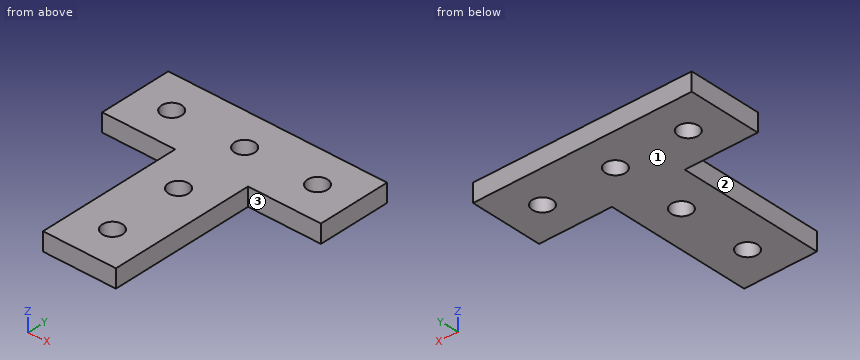
```python
from build123d import *

# Parameters (mm, degrees)
BOSS_EXTRUDE1_DEPTH = 6.35
SKETCH2_R           = 3.5
CUT_EXTRUDE1_DEPTH  = 7.35


with BuildPart() as part:
    # Sketch1 → Boss-Extrude1 (new body)
    with BuildSketch(Plane.XY):
        Polygon((12.7, 0), (-12.7, 0), (-12.7, 50.8), (-38.1, 50.8), (-38.1, 76.2), (38.1, 76.2), (38.1, 50.8), (12.7, 50.8), align=None)
    extrude(amount=BOSS_EXTRUDE1_DEPTH)

    # Sketch2 → Cut-Extrude1 (cut, through all)
    with BuildSketch(Plane.XY.offset(6.35)):
        with Locations((0, 63.5)):
            Circle(SKETCH2_R)
        with Locations((25.4, 63.5)):
            Circle(SKETCH2_R)
        with Locations((-25.4, 63.5)):
            Circle(SKETCH2_R)
        with Locations((0, 38.1)):
            Circle(SKETCH2_R)
        with Locations((0, 12.7)):
            Circle(SKETCH2_R)
    extrude(amount=-CUT_EXTRUDE1_DEPTH, mode=Mode.SUBTRACT)


solid = part.part
```
Read the model definition and answer for the solid it produces. Units are mm, in the model's axes. Face numbers are marked on the shaded views. A direction names the side the tool comes from. Coordinates: 2 decimals unless noted, no trailing zeros. Write each loop counter-clockwise with the first axis right and the second up, starting at its lowest first coordinate (ties: lowest second). Pieces come first, ordered by that corner, then holes. Notation, with made-up numbers: (-19.75, 43) -> (21.25, 43) arc R23 ccw to (21.25, 62) -> close; hole circle Ø5 at (-3.5, -34.5). An arc over 180 degrees is marked (long way). Answer as a JSON object with one key per item and string values.
Q1. Consider line 1 (Y direction, x = 0, z = 3.25); line 2 (Y direction, x = 25.4, z = 4.5); line 3 (X direction, y = 34.5, z = 3.75). Determine where each line is inside the solid, lowest interval first. Write a range as [from, to].
The answers:
{"line 1": "y = [0, 9.2], [16.2, 34.6], [41.6, 60], [67, 76.2]", "line 2": "y = [50.8, 60], [67, 76.2]", "line 3": "x = [-12.7, 12.7]"}
Q2. The part is cut by section B-B on y = 12.7. Give the vertices of the cut face in (x, z).
The answers:
{"outline": "(-12.7, 0) -> (-3.5, 0) -> (-3.5, 6.35) -> (-12.7, 6.35) -> close; (3.5, 0) -> (12.7, 0) -> (12.7, 6.35) -> (3.5, 6.35) -> close"}
Q3. The part is cut by section A-A on x = 25.4. Give the vertices of the cut face in (y, z).
The answers:
{"outline": "(50.8, 0) -> (60, 0) -> (60, 6.35) -> (50.8, 6.35) -> close; (67, 0) -> (76.2, 0) -> (76.2, 6.35) -> (67, 6.35) -> close"}
Q4. The part is cut by section D-D on y = 63.5. Give the vertices of the cut face in (x, z).
The answers:
{"outline": "(-38.1, 0) -> (-28.9, 0) -> (-28.9, 6.35) -> (-38.1, 6.35) -> close; (-21.9, 0) -> (-3.5, 0) -> (-3.5, 6.35) -> (-21.9, 6.35) -> close; (3.5, 0) -> (21.9, 0) -> (21.9, 6.35) -> (3.5, 6.35) -> close; (28.9, 0) -> (38.1, 0) -> (38.1, 6.35) -> (28.9, 6.35) -> close"}
Q5. Flat-ended cylindrical pins translate along their axes: pin 1 Ø6.5 at (x, y) = (0, 12.7) entering from +Z; pin 2 Ø1.9 at (y, z) = (26.5, 3) entering from -X; pin 3 Ø1.9 at (x, z) = (28.5, 4.5) entering from -Y; pin 4 Ø1.9 at (y, z) = (28, 2) entering from +X. Find the tip coordinate at first contact, or state that the pin passes through.
The answers:
{"pin 1": "passes through", "pin 2": "stops at x = -12.7", "pin 3": "stops at y = 50.8", "pin 4": "stops at x = 12.7"}
Q6. The part is cut by section C-C on z = 4.75. Give the vertices of the cut face in (x, y).
The answers:
{"outline": "(-38.1, 50.8) -> (-12.7, 50.8) -> (-12.7, 0) -> (12.7, 0) -> (12.7, 50.8) -> (38.1, 50.8) -> (38.1, 76.2) -> (-38.1, 76.2) -> close; hole circle Ø7 at (-25.4, 63.5); hole circle Ø7 at (0, 12.7); hole circle Ø7 at (0, 38.1); hole circle Ø7 at (0, 63.5); hole circle Ø7 at (25.4, 63.5)"}
Q7. A tool of negligible diameter and unlimited length cuts with its end or side. For the marked faces 1, 2 and 3, from which of +Z, -Z, +X, -X, +Y, -Y can it reach the whole face along a straight path? Write none if from no direction.
The answers:
{"face 1": "-Z, +X, -X, +Y, -Y", "face 2": "+Z, -Z, -X, -Y", "face 3": "+Z, -Z, +X, -Y"}
